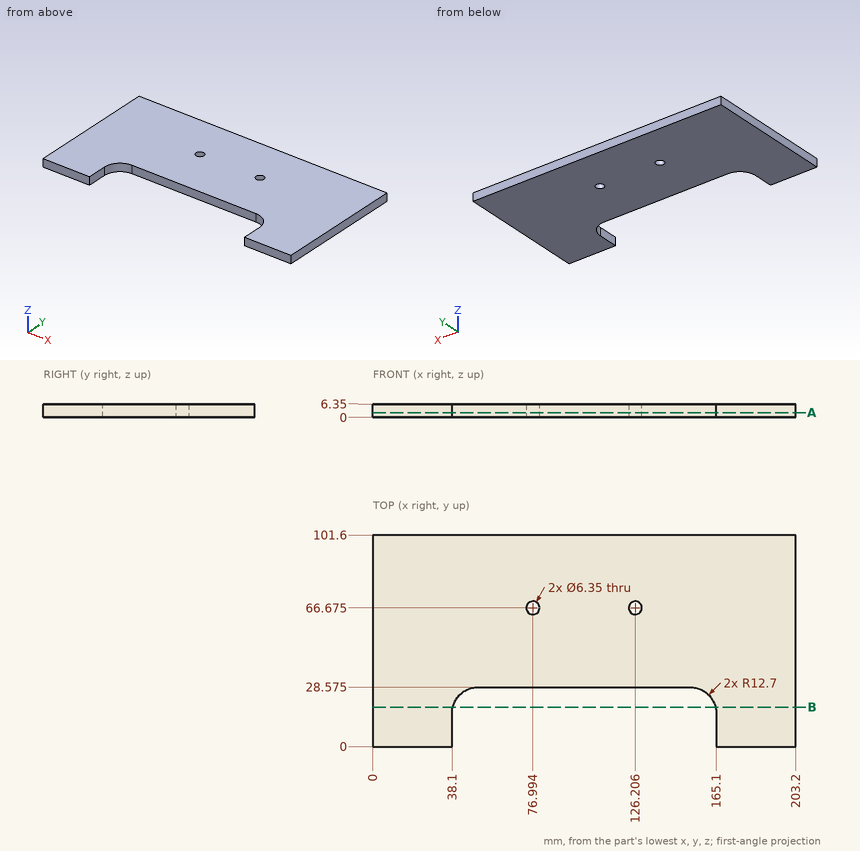
Verification items for this drawing (mm, ordinates from the low corner). Round coordinates to 2 decimals unless told otherwise and drop trailing zeros. Order: outer loops, then holes, each group sorted by start corner. A loop starts at its lowest first (then second) coordinate and runs counter-clockwise, first axis right, second up. Notation, with made-up numbers: (66.25, 32) -> (110.25, 32) arc R9 ccw to (110.25, 48) -> close; hole circle Ø6 at (-3.5, 41.5). An arc over 180 degrees is marked (long way). Use one line per item in the form item = value.
1. Cross-section at B-B, the plane y = 19. Enter the section's corners in (x, z).
Working result:
outline = (0, 0) -> (38.49, 0) -> (38.49, 6.35) -> (0, 6.35) -> close; (164.71, 0) -> (203.2, 0) -> (203.2, 6.35) -> (164.71, 6.35) -> close
2. Cross-section at A-A, the plane z = 2.25. Count the separate pieces of the cut face and the enclosed holes in it, plus the area to 3 significant figures.
Working result:
separate_pieces = 1
enclosed_holes = 2
area = 17,000 mm^2
3. Go/stop test with flat-tipped pins: pin 1 (3 mm diameter, centred on x = 118, z = 3.5, fed in from -Y) (3 decimals); pin 2 (10 mm diameter, centred on x = 76.99, y = 66.68, fed in from -Z). Record where each tip stops, or that it passes through.
Working result:
pin_1 = 28.575
pin_2 = 0
4. Scan lines: line 1 along X through (y, z) = (66.5, 2.5); line 2 along X through (y, z) = (7, 6); line 3 along Y through (x, z) = (120, 4.5) (1 decimal). Record each from-to range of solid material in increasing order. Write a range as from..to.
Working result:
line_1 = 0..73.82, 80.16..123.04, 129.38..203.2
line_2 = 0..38.1, 165.1..203.2
line_3 = 28.6..101.6
